from build123d import *

# Parameters (mm, degrees)
SKETCH1_R           = 6.35
BOSS_EXTRUDE1_DEPTH = 421.64
SKETCH2_R           = 10.795
BOSS_EXTRUDE2_DEPTH = 421.64
SKETCH3_R           = 25.4
SKETCH3_R_2         = 6.35
CUT_EXTRUDE1_DEPTH  = 52.324
CUT_EXTRUDE2_START  = -57.658
SKETCH4_R           = 25.4
SKETCH4_R_2         = 6.35
CUT_EXTRUDE2_DEPTH  = 57.658
CHAMFER1_SIZE       = 6.35
SKETCH5_R           = 15.875
CUT_EXTRUDE3_DEPTH  = 212.372033273
CUT_EXTRUDE4_DEPTH  = 19.304


with BuildPart() as part:
    # Sketch1 → Boss-Extrude1 (new body)
    with BuildSketch(Plane(origin=(0, 0, 0), x_dir=(1, 0, 0), z_dir=(0, 1, 0))):
        with Locations(Location((0, 0, 0), (0, 0, 270))):
            Circle(SKETCH1_R)
    extrude(amount=BOSS_EXTRUDE1_DEPTH)

    # Sketch2 → Boss-Extrude2 (add)
    with BuildSketch(Plane(origin=(0, 0, 0), x_dir=(-1, 0, 0), z_dir=(0, -1, 0))):
        with Locations(Location((0, 0, 0), (0, 0, 90))):
            Circle(SKETCH2_R)
    extrude(amount=-BOSS_EXTRUDE2_DEPTH)

    # Sketch3 → Cut-Extrude1 (cut)
    with BuildSketch(Plane.XZ):
        Circle(SKETCH3_R)
        with Locations(Location((0, 0, 0), (0, 0, 270))):
            Circle(SKETCH3_R_2, mode=Mode.SUBTRACT)
    extrude(amount=-CUT_EXTRUDE1_DEPTH, mode=Mode.SUBTRACT)

    # Sketch4 → Cut-Extrude2 (cut)
    with BuildSketch(Plane(origin=(0, 421.64, 0), x_dir=(1, 0, 0), z_dir=(0, 1, 0)).offset(CUT_EXTRUDE2_START)):
        Circle(SKETCH4_R)
        with Locations(Location((0, 0, 0), (0, 0, 90))):
            Circle(SKETCH4_R_2, mode=Mode.SUBTRACT)
    extrude(amount=CUT_EXTRUDE2_DEPTH, mode=Mode.SUBTRACT)

    # Chamfer1
    # the kernel refuses this chamfer: 6.35 mm, written as the material it takes off along each edge
    with BuildSketch(Plane(origin=(0, 52.324, 0), x_dir=(0, 0, -1), z_dir=(-1, 0, 0))) as chamfer1_piece_1_section:
        Polygon((10.795, -CHAMFER1_SIZE), (10.795 - CHAMFER1_SIZE, 0), (10.795, 0), align=None)
    chamfer1_piece_1 = revolve(axis=Axis((0, 52.324, 0), (0, -1, 0)), mode=Mode.PRIVATE)
    chamfer1_piece_1 = chamfer1_piece_1 - Plane(origin=(0, 56.4676015, 0), x_dir=(0, 0, -1), z_dir=(0, -1, 0)) * Cylinder(6.35, 44, mode=Mode.PRIVATE)
    add(chamfer1_piece_1, mode=Mode.SUBTRACT)
    with BuildSketch(Plane(origin=(0, 363.982, 0), x_dir=(0, 0, -1), z_dir=(-1, 0, 0))) as chamfer1_piece_2_section:
        Polygon((10.795, CHAMFER1_SIZE), (10.795 - CHAMFER1_SIZE, 0), (10.795, 0), align=None)
    chamfer1_piece_2 = revolve(axis=Axis((0, 363.982, 0), (0, -1, 0)), mode=Mode.PRIVATE)
    chamfer1_piece_2 = chamfer1_piece_2 - Plane(origin=(0, 359.8383985, 0), x_dir=(0, 0, -1), z_dir=(0, -1, 0)) * Cylinder(6.35, 44, mode=Mode.PRIVATE)
    add(chamfer1_piece_2, mode=Mode.SUBTRACT)

    # Sketch5 → Cut-Extrude3 (cut, through all)
    with BuildSketch(Plane(origin=(0, 210.82, 0), x_dir=(1, 0, 0), z_dir=(0, 1, 0))):
        Circle(SKETCH5_R)
    extrude(amount=-CUT_EXTRUDE3_DEPTH, mode=Mode.SUBTRACT)

    # Sketch6 → Cut-Extrude4 (cut)
    with BuildSketch(Plane(origin=(0, 210.82, 0), x_dir=(-1, 0, 0), z_dir=(0, -1, 0))):
        Polygon((-5.054761839, -3.255740788), (0.292173311, -6.005422557), (5.346935151, -2.749681769), (5.054761839, 3.255740788), (-0.292173311, 6.005422557), (-5.346935151, 2.749681769), align=None)
    extrude(amount=-CUT_EXTRUDE4_DEPTH, mode=Mode.SUBTRACT)


solid = part.part
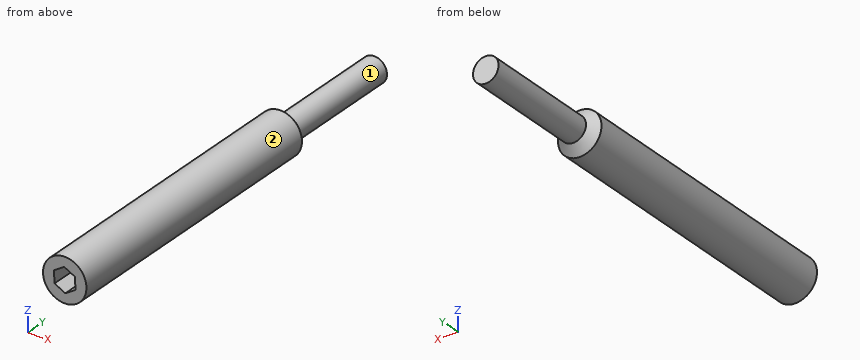
Work out the finished part from the listing and answer in its coordinate system (mm). Face numbers are marked on the shaded views. A direction names the side the tool comes from. Coordinates: 2 decimals unless noted, no trailing zeros. Order: outer loops, then holes, each group sorted by start corner. A loop starts at its lowest first (then second) coordinate and runs counter-clockwise, first axis right, second up. Notation, with made-up numbers: (-37, 42) - (-25, 42) arc R23 cw to (-25, 65) - close; hole circle Ø5 at (-32, -40). An arc over 180 degrees is marked (long way). Put each result on its own line as item: value. Start each with the question number.
1) For the marked faces 1 and 2, determine the directions among +Z, -Z, +X, -X, +Y, -Y from which every point of the face is accessible in a straight line to the end or side of a thin tool.
2) Flat-ended cylindrical pins translate along their axes: pin 1 (4 mm diameter, centred on y = 318, z = -5.5, fed in from -X); pin 2 (4 mm diameter, centred on y = 377, z = -2, fed in from +X); pin 3 (5 mm diameter, centred on x = 5.5, y = 250.5, fed in from -Z). Find the tip coordinate at first contact, or state that the pin passes through.
3) Find section B-B (y = 264). Give the vertices of the cut face in (x, z) (3 decimals).
4) Find section A-A (z = 0). Give the vertices of the cut face in (x, y) (3 decimals).
5) Find the intervals of material crossed by line 1 (Y direction, x = 1.25, z = 2); line 2 (Z direction, x = -7.25, y = 276.5); line 3 (Z direction, x = -6.75, y = 318), in increasing order. Write a range as from..to.
Results list:
1. face 1: +Y
1. face 2: +Y, -Y
2. pin 1: stops at x = -10.21
2. pin 2: stops at x = 6.35
2. pin 3: stops at z = -10.37
3. outline: circle Ø21.59 at (0, 0)
4. outline: (-10.795, 210.82) - (-5.213, 210.82) - (-5.213, 230.124) - (5.213, 230.124) - (5.213, 210.82) - (10.795, 210.82) - (10.795, 357.632) - (6.35, 362.077) - (6.35, 421.64) - (-6.35, 421.64) - (-6.35, 362.077) - (-10.795, 357.632) - close
5. line 1: y = 230.12..421.64
5. line 2: z = -8..8
5. line 3: z = -8.42..8.42
